```python
from build123d import *

# Parameters (mm, degrees)
F0_R            = 63.5
F0_R_2          = 37.3126
F1_DEPTH        = 67.231133
F5_DEPTH        = 67.231133
F5_COPIES_COUNT = 9
F6_COUNT        = 9
F6_ANGLE        = 320


# Not quite as in the source:
# - a pattern or mirror of a feature is missing from the dataset's text; its kind, count and spacing are read off the source's solid


with BuildPart() as f1:
    # F0 (on Top) → F1 (new body)
    with BuildSketch(Plane.XY):
        Circle(F0_R)
        Circle(F0_R_2, mode=Mode.SUBTRACT)
    extrude(amount=F1_DEPTH)

    # F2 (on Front) → F3 (revolve, cut)
    with BuildSketch(Plane.XZ):
        Polygon((43.6626, 110.893733), (43.6626, 67.231133), (63.5, 12.7), (63.5, 0), (107.1626, 0), (107.1626, 110.893733), align=None)
    revolve(axis=Axis((0, 0, 67.231133), (0, 0, 1)), mode=Mode.SUBTRACT)

    # F4 (on face) → F5 (cut, through all)
    with BuildSketch(Plane(origin=(0, 0, 0), x_dir=(1, 0, 0), z_dir=(0, 0, -1))):
        with BuildLine():
            ThreePointArc((-37.0996847558, -11.6974856713), (-38.9001, 0), (-37.0996847558, 11.6974856713))
            Line((-37.0996847558, 11.6974856713), (-60.2295137998, 20.116054967))
            ThreePointArc((-60.2295137998, 20.116054967), (-63.5, 0), (-60.2295137998, -20.116054967))
            Line((-60.2295137998, -20.116054967), (-37.0996847558, -11.6974856713))
        make_face()
    f5 = extrude(amount=-F5_DEPTH, mode=Mode.SUBTRACT)

    # F5_copies: F5 ×9 about axis
    f5_copies_axis = Axis((0, 0, 0), (0, 0, 1))
    for i in range(1, F5_COPIES_COUNT):
        add(f5.rotate(f5_copies_axis, i * 360 / F5_COPIES_COUNT), mode=Mode.SUBTRACT)

    # F6: F5 ×9 about axis
    f6_axis = Axis((0, 0, 67.231133), (0, 0, -1))
    for i in range(1, F6_COUNT):
        add(f5.rotate(f6_axis, i * F6_ANGLE / (F6_COUNT - 1)), mode=Mode.SUBTRACT)


solid = f1.part
```
Design review of the part built by this model. Coordinates are the model's own, in mm. A direction names the side the tool comes from. Give positions to 0.01 mm unless a question says otherwise; leave off trailing zeros. Write each loop counter-clockwise with the first axis right and the second up, starting at its lowest first coordinate (ties: lowest second). Pieces come first, ordered by that corner, then holes. Notation, with made-up numbers: (84, 32.5) - (133, 32.5) arc R23 cw to (133, 40.5) - close; hole circle Ø10 at (68, 24.25). An arc over 180 degrees is marked (long way). Return JSON: item names as keys, results as strings. Group by question number.
(1) Machinability: for faces 4 (the flat face through (-44.77, 18.1, 25.67)), 5 (the flat face through (-25.773, 41.247, 25.675)), 6 (the flat face through (35.88, -32.32, 25.67)), which of the approach directions +Z, -Z, +X, -X, +Y, -Y give a long, thin tool a straight path to every point of the face, cutting with its end or side? Answer none if there is none.
(2) Insertion check: pin 1 (10 mm diameter, centred on y = -21, z = 10, fed in from +X); pin 2 (4 mm diameter, centred on y = 40, z = 16, fed in from +X); pin 3 (10 mm diameter, centred on y = 37.5, z = 36, fed in from -X). Each pin has a flat end and moves straight along its axis. Give the tip position at first contact, or say it passes through.
(3) We need section B-B, the plane x = 0. Give the boundary of the cut face in (y, z).
(4) To check wall thickness, follow probe 1 along Y at (x, z) = (0, 30); probe 2 along X at (y, z) = (-29, 27.5); probe 3 along Y at (x, z) = (31, 27.5). State the ranges of each line that lie inside material, in increasing order.
(5) We need section A-A, the plane y = 0. Give the boundary of the cut face in (x, z), then the cut area to 3 significant figures.
(6) We need section C-C, the plane x = -15.5. Give the boundary of the cut face in (y, z).
(7) Mouldability with a two-part tool opening along X and no side actions: class faces 1 (the cylindrical face through (-38.9, 0.2, 33.1)), 2 (the flat face through (49, 1.697, 26)), 3 (the flat face through (6.71, -47.82, 25.67)) as +X half, -X half, draft (parallel to the pull), parting line (faces both ways), or undercut.
Reported:
{
 "1": {"face 4": "+Z, -Z, +Y", "face 5": "+Z, -Z, -X", "face 6": "+Z, -Z, -Y"},
 "2": {"pin 1": "stops at x = 35.46", "pin 2": "stops at x = 49.3", "pin 3": "stops at x = -26.5"},
 "3": {"outline": "(-38.9, 0) - (-37.31, 0) - (-37.31, 67.23) - (-38.9, 67.23) - close; (37.31, 0) - (38.9, 0) - (38.9, 67.23) - (37.31, 67.23) - close"},
 "4": {"probe 1": "y = -38.9 to -37.31, 37.31 to 38.9", "probe 2": "x = -25.93 to -23.48, 23.48 to 25.93, 31.92 to 37.2", "probe 3": "y = -28.23 to -23.8, -23.5 to -20.77, 20.77 to 23.5, 23.8 to 28.23"},
 "5": {"outline": "(-38.9, 0) - (-37.31, 0) - (-37.31, 67.23) - (-38.9, 67.23) - close; (37.31, 0) - (63.5, 0) - (63.5, 12.7) - (43.66, 67.23) - (37.31, 67.23) - close", "area": "1,330 mm2"},
 "6": {"outline": "(-35.68, 0) - (-33.94, 0) - (-33.94, 67.23) - (-35.68, 67.23) - close; (33.94, 0) - (35.68, 0) - (35.68, 67.23) - (33.94, 67.23) - close"},
 "7": {"face 1": "-X half", "face 2": "draft", "face 3": "undercut"}
}
